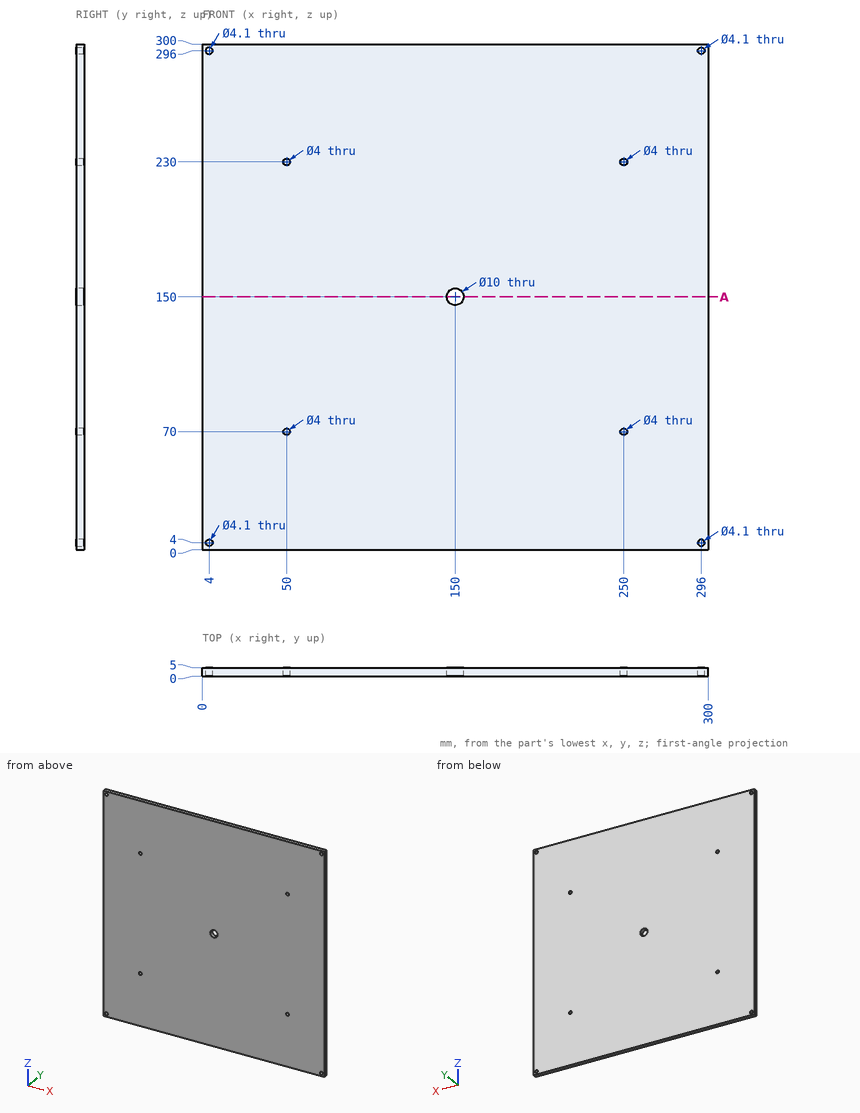
Drawing for the job (mm, zero at the part's lowest x, y, z). Give positions to 0.01 mm unless a question says otherwise; leave off trailing zeros. Loops run counter-clockwise (first coordinate to the right, second up) from the corner with the lowest first, then second, coordinate; pieces in that order, holes last.
(1) Drill centre lines: line 1 along X through (y, z) = (1.55, 4); line 2 along X through (y, z) = (3.4, 230); line 3 along X through (y, z) = (2.25, 150). Where is each one in solid material? Low to high.
Return value:
line 1: x = 0 to 1.95, 6.05 to 293.95, 298.05 to 300
line 2: x = 0 to 48, 52 to 248, 252 to 300
line 3: x = 0 to 145, 155 to 300
(2) Band-saw the part on A-A (z = 150). Write the cut outline in (x, y), and give its area (3 significant figures).
Return value:
outline: (0, 0) - (145, 0) - (145, 5) - (0, 5) - close; (155, 0) - (300, 0) - (300, 5) - (155, 5) - close
area: 1,450 mm2
(3) Pin check, flat tip, straight feed: pin 1 (3.5 mm diameter, centred on x = 296, z = 4, fed in from -Y) (3 decimals). Stop position of the tip, or through.
Return value:
pin 1: passes through
